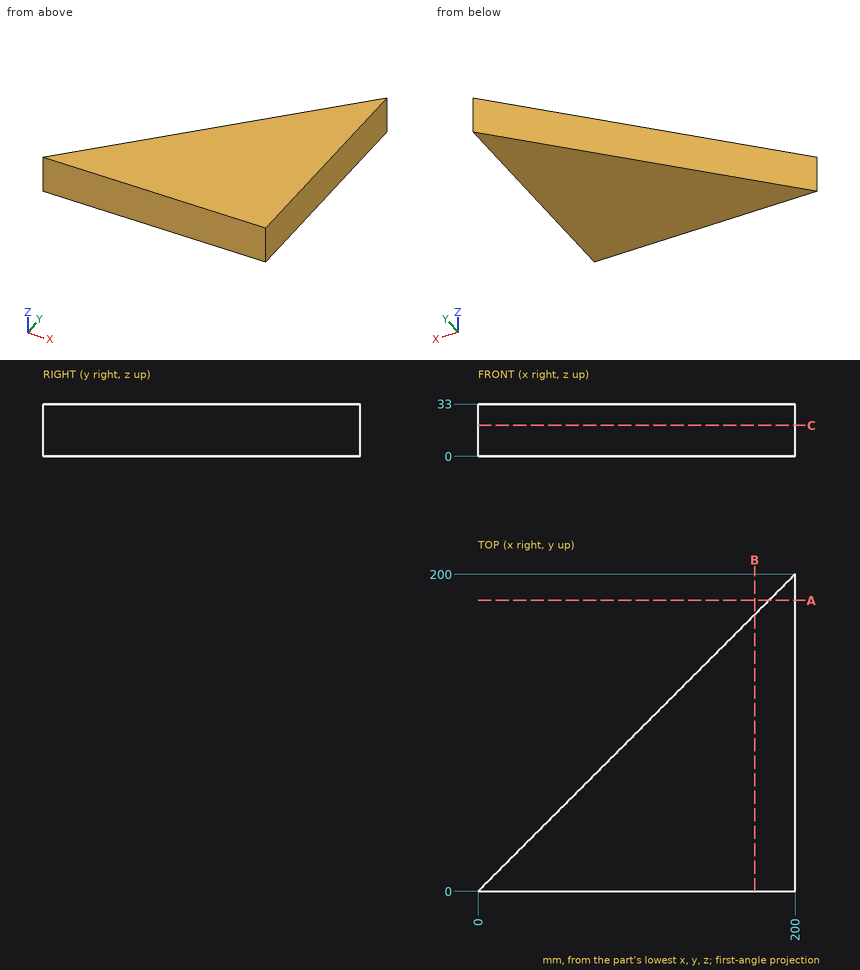
Here's the drawing with two shaded views (mm, measured from the low corner). I have some questions. Give positions to 0.01 mm unless a question says otherwise; leave off trailing zeros. Order: outer loops, then holes, each group sorted by start corner. A loop starts at its lowest first (then second) coordinate and runs counter-clockwise, first axis right, second up.
Q1. If I drill on line 1 along X through (y, z) = (34, 17); line 2 along Y through (x, z) = (131.5, 9); line 3 along Y through (x, z) = (52, 6.5), over which ranges is the centre line in solid material (lowest first)?
Q2. Suppose I cut it at C-C, the plane z = 19.5. Write out the boundary of the cut face in (x, y).
Q3. Suppose I cut it at B-B, the plane x = 174.5. Write out the boundary of the cut face in (y, z), and give its area (3 significant figures).
Q4. Suppose I cut it at A-A, the plane y = 183.5. Write out the boundary of the cut face in (x, z).
Solution:
1. line 1: x = 34 to 200
1. line 2: y = 0 to 131.5
1. line 3: y = 0 to 52
2. outline: (0, 0) - (200, 0) - (200, 200) - close
3. outline: (0, 0) - (174.5, 0) - (174.5, 33) - (0, 33) - close
3. area: 5,760 mm2
4. outline: (183.5, 0) - (200, 0) - (200, 33) - (183.5, 33) - close
